```python
from build123d import *

# Parameters (mm, degrees)
F1_DEPTH = 23.114
F2_W     = 30.988
F2_H     = 94.282678
F3_DEPTH = 86.36


with BuildPart() as f1:
    # F0 (on Right) → F1 (new body, symmetric)
    with BuildSketch(Plane.YZ):
        Polygon((18.332004, 56.31125), (-47.292158, 56.31125), (-3.433616, -37.281614), (38.789531, -37.281614), align=None)
    extrude(amount=F1_DEPTH, both=True)

    # F2 (on face) → F3 (cut)
    with BuildSketch(Plane(origin=(0, 0, -37.281614), x_dir=(1, 0, 0), z_dir=(0, 0, -1))):
        with Locations((0, 3.863558)):
            Rectangle(F2_W, F2_H)
    extrude(amount=-F3_DEPTH, mode=Mode.SUBTRACT)


solid = f1.part
```
Work out the finished part from the listing and answer in its coordinate system (mm). A direction names the side the tool comes from. Give positions to 0.01 mm unless a question says otherwise; leave off trailing zeros. Loops run counter-clockwise (first coordinate to the right, second up) from the corner with the lowest first, then second, coordinate; pieces in that order, holes last. Notation, with made-up numbers: (53, 17) -> (72, 17) arc R19 ccw to (72, 33) -> close; hole circle Ø5 at (24.25, -36.5). An arc over 180 degrees is marked (long way). Put each result on its own line as item: value. Start each with the question number.
Item 1: The part is cut by section D-D (x = 20). Give the vertices of the cut face in (y, z), then the cut area to 3 significant figures.
Item 2: The part is cut by section C-C (y = 6.5). Give the vertices of the cut face in (x, z), then the cut area to 3 significant figures.
Item 3: The part is cut by section B-B (y = 22). Give the vertices of the cut face in (x, z), then the cut area to 3 significant figures.
Item 4: Which of the six approach directions +Z, -Z, +X, -X, +Y, -Y give full straight-line access (tool end or side, diameter ignored) to faces 1 (the face through (-15.494, -2, 5)), 2 (the face through (-19, 17, -37.282))?
Item 5: This flat-tipped pin is pushed along its axis until it touches: P1, Ø3, axis at x = -16.5, z = -9.5, coming from the -Y side. Where does it stop, or does it pass through?
Item 6: The mould has two halves that part along X. Classify faces 3 (the face through (0, -12, 49.078)), 4 (the face through (-23.114, 5, 10)), 5 (the face through (15.733, -30.543, 20.569)): released by +X, released by -X, zero draft, split by the parting line, or undercut.
Item 7: Find the intervals of material crossed by L1, parallel to X at y = 14.5, z = 10; L2, parallel to Z at x = 2, y = -24.5; L3, parallel to Y at x = 17.5, z = -16, in increasing order. Write a range as [from, to].
Item 8: The part is cut by section A-A (z = -23.5). Give the vertices of the cut face in (x, y).
Answers below:
1. outline: (-47.29, 56.31) -> (-3.43, -37.28) -> (38.79, -37.28) -> (18.33, 56.31) -> close
1. area: 5,050 mm2
2. outline: (-23.11, -37.28) -> (-15.49, -37.28) -> (-15.49, 49.08) -> (15.49, 49.08) -> (15.49, -37.28) -> (23.11, -37.28) -> (23.11, 56.31) -> (-23.11, 56.31) -> close
2. area: 1,650 mm2
3. outline: (-23.11, -37.28) -> (-15.49, -37.28) -> (-15.49, 39.53) -> (-23.11, 39.53) -> close; (15.49, -37.28) -> (23.11, -37.28) -> (23.11, 39.53) -> (15.49, 39.53) -> close
3. area: 1,170 mm2
4. face 1: -Z, +Y, -Y
4. face 2: -Z, +X, -X, +Y, -Y
5. P1: y = -17.16
6. face 3: undercut
6. face 4: released by -X
6. face 5: zero draft
7. L1: [-23.11, -15.49], [15.49, 23.11]
7. L2: [49.08, 56.31]
7. L3: [-13.41, 34.14]
8. outline: (-23.11, -9.89) -> (-15.49, -9.89) -> (-15.49, 35.78) -> (-23.11, 35.78) -> close; (15.49, -9.89) -> (23.11, -9.89) -> (23.11, 35.78) -> (15.49, 35.78) -> close
